Source: three-view drawing plus pictorial views. Frame: mm from the lowest corner of the part. Give positions to 0.01 mm unless a question says otherwise; leave off trailing zeros. Order: outer loops, then holes, each group sorted by start corner. A loop starts at its lowest first (then second) coordinate and runs counter-clockwise, first axis right, second up. Notation, with made-up numbers: (-28.75, -3) - (7.25, -3) arc R19 ccw to (7.25, 16) - close; hole circle Ø10 at (42.25, -39). An arc over 180 degrees is marked (long way). Answer in a Markdown table with one row per item. Add a question column.
1. Contact query for flat-ended pins moving along their axis: pin 1 (2.5 mm diameter, centred on x = 6, z = 21.05, fed in from +Y); pin 2 (1.8 mm diameter, centred on x = 23.4, z = 21.05, fed in from +Y). Output: stop coordinate, or through.
2. Section query B-B on z = 3.05. Return loops of the section in (x, y).
3. Ray query, line 1 (Z direction, x = 6, y = 1.75); line 2 (X direction, y = 0.8, z = 21.05). Return the intervals inside material, ascending. Write a range as [from, to].
4. Section query C-C on y = 1.75. Return loops of the section in (x, z), and give its area (3 significant figures).
5. Section query A-A on x = 23.4. Return loops of the section in (y, z), and give its area (4 significant figures).
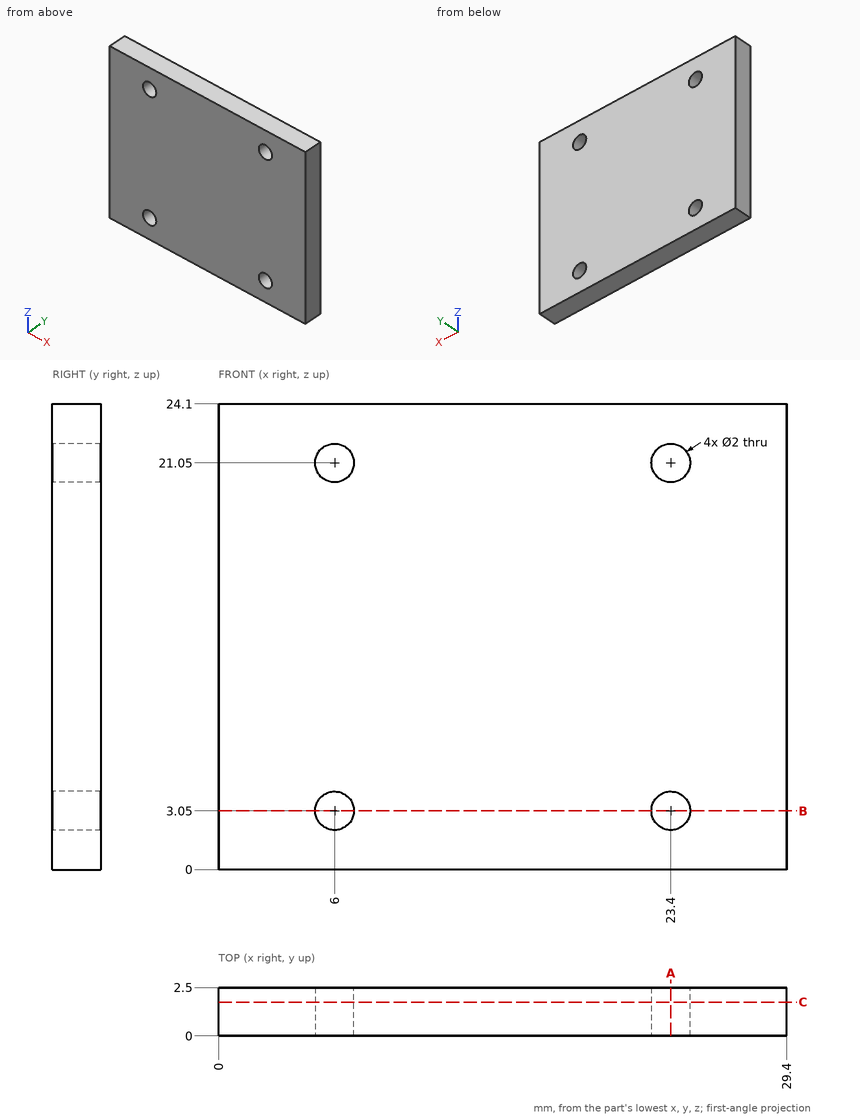
Answer:
| question | item | result |
|---|---|---|
| 1 | pin 1 | stops at y = 2.5 |
| 1 | pin 2 | passes through |
| 2 | outline | (0, 0) - (5, 0) - (5, 2.5) - (0, 2.5) - close; (7, 0) - (22.4, 0) - (22.4, 2.5) - (7, 2.5) - close; (24.4, 0) - (29.4, 0) - (29.4, 2.5) - (24.4, 2.5) - close |
| 3 | line 1 | z = [0, 2.05], [4.05, 20.05], [22.05, 24.1] |
| 3 | line 2 | x = [0, 5], [7, 22.4], [24.4, 29.4] |
| 4 | outline | (0, 0) - (29.4, 0) - (29.4, 24.1) - (0, 24.1) - close; hole circle Ø2 at (6, 3.05); hole circle Ø2 at (6, 21.05); hole circle Ø2 at (23.4, 3.05); hole circle Ø2 at (23.4, 21.05) |
| 4 | area | 696 mm² |
| 5 | outline | (0, 0) - (2.5, 0) - (2.5, 2.05) - (0, 2.05) - close; (0, 4.05) - (2.5, 4.05) - (2.5, 20.05) - (0, 20.05) - close; (0, 22.05) - (2.5, 22.05) - (2.5, 24.1) - (0, 24.1) - close |
| 5 | area | 50.25 mm² |
